Model file for the job. Use its own axes, mm. Face numbers are marked on the shaded views. A direction names the side the tool comes from. Round coordinates to 2 decimals unless told otherwise and drop trailing zeros. Order: outer loops, then holes, each group sorted by start corner. A loop starts at its lowest first (then second) coordinate and runs counter-clockwise, first axis right, second up. Notation, with made-up numbers: (30.5, -7) - (63.5, -7) arc R13 cw to (63.5, -1) - close; hole circle Ø8 at (18, 23). An arc over 180 degrees is marked (long way). Put each result on its own line as item: value. Start each with the question number.
Item 1: Saw through at A-A on z = 23. List the corners of the cut face in (x, y), plus the area to 3 significant figures.
Item 2: Which spindle directions (+Z, -Z, +X, -X, +Y, -Y) get a long thin tool onto all of the face, cutting with end or side? Do the marked faces 1 and 2. Say none if no direction does.
Item 3: Saw through at B-B on x = 1.25. List the corners of the cut face in (y, z), plus the area to 3 significant figures.
Item 4: Saw through at C-C on z = 15. List the corners of the cut face in (x, y), plus the area to 3 significant figures.
Item 5: Pin check, flat tips, straight feed: pin 1 Ø2.5 at (x, z) = (6.62, 23) entering from -Y; pin 2 Ø5 at (x, z) = (-6.71, 23) entering from -Y; pin 3 Ø1 at (x, y) = (7.5, 7.5) entering from +Z. Stop position of each tip, or through.
Item 6: Probe probe 1 along X at (y, z) = (15.3, 23); probe 2 along X at (y, z) = (15.2, 15); probe 3 along Z at (x, y) = (-4.75, 0). List the from-to ranges inside material, lowest first.
Item 7: Saw through at D-D on y = 11. List the corners of the cut face in (x, z), plus the area to 3 significant figures.
```python
from build123d import *

# Parameters (mm, degrees)
ESBO_O1_R                = 3.45
ESBO_O1_R_2              = 1.15
RESSALTO_EXTRUS_O2_DEPTH = 2
ESBO_O2_W                = 25
ESBO_O2_H                = 2
RESSALTO_EXTRUS_O3_DEPTH = 28
ESBO_O3_R                = 5
ESBO_O3_R_2              = 2
CORTE_EXTRUS_O1_DEPTH    = 2
FILETE1_R                = 3
FILETE2_R                = 3


with BuildPart() as part:
    # Esboço1 → Ressalto-extrusão2 (new body)
    with BuildSketch(Plane.XY):
        with BuildLine():
            Line((12.456898993, -4), (12.456898993, 16.5))
            Line((12.456898993, 16.5), (-12.543101007, 16.5))
            Line((-12.543101007, 16.5), (-12.543101007, -4))
            ThreePointArc((-12.543101007, -4), (-0.043101007, -16.5), (12.456898993, -4))
        make_face()
        with Locations((-0.043101007, -4)):
            Circle(ESBO_O1_R, mode=Mode.SUBTRACT)
        with Locations((8.706898993, -4)):
            Circle(ESBO_O1_R_2, mode=Mode.SUBTRACT)
        with Locations((-8.793101007, -4)):
            Circle(ESBO_O1_R_2, mode=Mode.SUBTRACT)
    extrude(amount=RESSALTO_EXTRUS_O2_DEPTH)

    # Esboço2 → Ressalto-extrusão3 (add)
    with BuildSketch(Plane.XY.offset(2)):
        with Locations((-0.043101007, 15.5)):
            Rectangle(ESBO_O2_W, ESBO_O2_H)
    extrude(amount=RESSALTO_EXTRUS_O3_DEPTH)

    # Esboço3 → Corte-extrusão1 (cut)
    with BuildSketch(Plane.XZ.offset(-14.5)):
        with Locations(Location((-0.043101007, 15, 0), (0, 0, 270))):
            Circle(ESBO_O3_R)
        with Locations(Location((-6.709767674, 7, 0), (0, 0, 270))):
            Circle(ESBO_O3_R_2)
        with Locations(Location((6.623565659, 7, 0), (0, 0, 90))):
            Circle(ESBO_O3_R_2)
        with Locations(Location((6.623565659, 23, 0), (0, 0, 270))):
            Circle(ESBO_O3_R_2)
        with Locations(Location((-6.709767674, 23, 0), (0, 0, 90))):
            Circle(ESBO_O3_R_2)
    extrude(amount=-CORTE_EXTRUS_O1_DEPTH, mode=Mode.SUBTRACT)

    # Filete1
    filete1_edges = [part.edges().sort_by_distance(p)[0] for p in [
        (12.456898993, 15.5, 30),
    ]]
    fillet(filete1_edges, radius=FILETE1_R)

    # Filete2
    filete2_edges = [part.edges().sort_by_distance(p)[0] for p in [
        (-12.543101007, 15.5, 30),
    ]]
    fillet(filete2_edges, radius=FILETE2_R)


solid = part.part
```
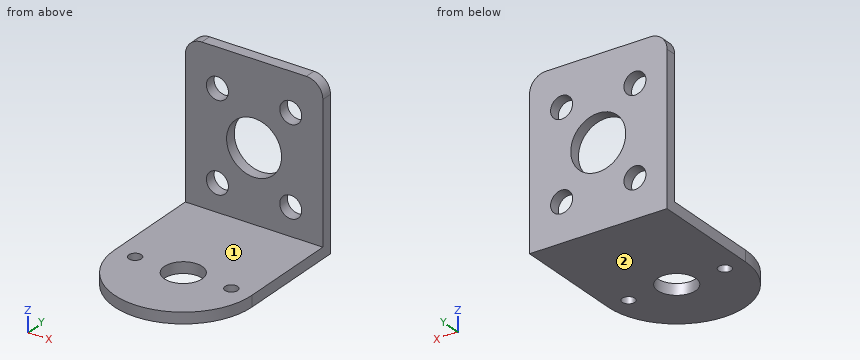
Results found:
1. outline: (-12.54, 14.5) - (-8.71, 14.5) - (-8.71, 16.5) - (-12.54, 16.5) - close; (-4.71, 14.5) - (4.62, 14.5) - (4.62, 16.5) - (-4.71, 16.5) - close; (8.62, 14.5) - (12.46, 14.5) - (12.46, 16.5) - (8.62, 16.5) - close
1. area: 34.0 mm²
2. face 1: +Z, +X, -X, -Y
2. face 2: -Z, +X, -X, +Y, -Y
3. outline: (-16.43, 0) - (-7.2, 0) - (-7.2, 2) - (-16.43, 2) - close; (-0.8, 0) - (16.5, 0) - (16.5, 10.17) - (14.5, 10.17) - (14.5, 2) - (-0.8, 2) - close; (14.5, 19.83) - (16.5, 19.83) - (16.5, 30) - (14.5, 30) - close
3. area: 89.8 mm²
4. outline: (-12.54, 14.5) - (-5.04, 14.5) - (-5.04, 16.5) - (-12.54, 16.5) - close; (4.96, 14.5) - (12.46, 14.5) - (12.46, 16.5) - (4.96, 16.5) - close
4. area: 30.0 mm²
5. pin 1: passes through
5. pin 2: stops at y = 14.5
5. pin 3: stops at z = 2
6. probe 1: x = -12.54 to -8.71, -4.71 to 4.62, 8.62 to 12.46
6. probe 2: x = -12.54 to -5.04, 4.96 to 12.46
6. probe 3: z = 0 to 2
7. outline: (-12.54, 0) - (12.46, 0) - (12.46, 2) - (-12.54, 2) - close
7. area: 50.0 mm²
